```python
from build123d import *

# Parameters (mm, degrees)
SKETCH1_R           = 7.5
BOSS_EXTRUDE1_DEPTH = 230
SKETCH2_R           = 10
BOSS_EXTRUDE2_DEPTH = 5
SKETCH3_R           = 7.5
BOSS_EXTRUDE3_DEPTH = 10
CUT_EXTRUDE1_DEPTH  = 80
EXTRUDE_THIN1_DEPTH = 1.5


with BuildPart() as part:
    # Sketch1 → Boss-Extrude1 (new body)
    with BuildSketch(Plane.XY):
        Circle(SKETCH1_R)
    extrude(amount=BOSS_EXTRUDE1_DEPTH)

    # Sketch2 → Boss-Extrude2 (add)
    with BuildSketch(Plane.XY.offset(230)):
        Circle(SKETCH2_R)
    extrude(amount=BOSS_EXTRUDE2_DEPTH)

    # Sketch3 → Boss-Extrude3 (add)
    with BuildSketch(Plane.XY.offset(235)):
        Circle(SKETCH3_R)
    extrude(amount=BOSS_EXTRUDE3_DEPTH)

    # Sketch4 → Cut-Extrude1 (cut)
    with BuildSketch(Plane(origin=(0, 0, 0), x_dir=(-1, 0, 0), z_dir=(0, 0, -1))):
        with BuildLine():
            Line((-6.5, 3.741657387), (-6.5, -3.741657387))
            ThreePointArc((-6.5, -3.741657387), (-7.5, 0), (-6.5, 3.741657387))
        make_face()
        with BuildLine():
            Line((6.5, 3.741657387), (6.5, -3.741657387))
            ThreePointArc((6.5, -3.741657387), (7.5, 0), (6.5, 3.741657387))
        make_face()
    extrude(amount=-CUT_EXTRUDE1_DEPTH, mode=Mode.SUBTRACT)

    # Sketch5 → Extrude-Thin1 (add, symmetric)
    with BuildSketch(Plane(origin=(0, 0, 0), x_dir=(1, 0, 0), z_dir=(0, 1, 0))):
        with BuildLine():
            Line((-6, -245), (-6, -248))
            ThreePointArc((-6, -248), (0, -254), (6, -248))
            Line((6, -248), (6, -245))
            Line((6, -245), (16, -245))
            Line((16, -245), (16, -248))
            ThreePointArc((16, -248), (0, -264), (-16, -248))
            Line((-16, -248), (-16, -245))
            Line((-16, -245), (-6, -245))
        make_face()
    extrude(amount=EXTRUDE_THIN1_DEPTH, both=True)


solid = part.part
```
Check sheet for the modelled part. Datum: model origin and axes. Units: mm. A direction names the side the tool comes from. Round coordinates to 2 decimals unless told otherwise and drop trailing zeros. Loops run counter-clockwise (first coordinate to the right, second up) from the corner with the lowest first, then second, coordinate; pieces in that order, holes last. Notation, with made-up numbers: M 67,-30 L 92,-30 A13 cw 92,-11 Z; hole C 64,59.5 d2. An arc over 180 degrees is marked long. Answer as a JSON object with one key per item and string values.
1. Scan lines: line 1 (Y direction, x = 0.5, z = 26); line 2 (X direction, y = -6.5, z = 218); line 3 (Z direction, x = 4.5, y = 2.5). Record each from-to range of solid material in increasing order.
Reply:
{"line 1": "y = -7.48 to 7.48", "line 2": "x = -3.74 to 3.74", "line 3": "z = 0 to 245"}
2. Section check B-B (z = 198). Record the boundary of the cut face in (x, y).
Reply:
{"outline": "C 0,0 d15"}
3. Gauge pin test, flat ends, axial feed: P1, Ø1, axis at x = 0.5, z = 225.5, coming from the +Y side; P2, Ø1, axis at x = -11, y = 3.5, coming from the +Z side; P3, Ø6, axis at y = 0, z = 36, coming from the +X side; P4, Ø3.5, axis at x = 10, y = 0.5, coming from the -Z side. Record the tip position at first contact, or that the pin passes through.
Reply:
{"P1": "stops at y = 7.5", "P2": "passes through", "P3": "stops at x = 6.5", "P4": "stops at z = 230"}
4. Access from +Z, -Z, +X, -X, +Y, -Y to the whole of each face (thin tool, end or side, straight path). Record for faces 1 (the flat face through (0.2, -1.5, 254.4)), 2 (the flat face through (-6.5, 0, 39)), 3 (the flat face through (6.5, 0, 39)), 4 (the flat face through (0.2, 1.5, 254.4)).
Reply:
{"face 1": "+Z, +X, -X, -Y", "face 2": "-Z, -X, +Y, -Y", "face 3": "-Z, +X, +Y, -Y", "face 4": "+Z, +X, -X, +Y"}
5. Mould release check, pull along X, two halves, no side actions. Record for faces 5 (the flat face through (4, 7, 230)), 6 (the cylindrical face through (-7.493, 0.33, 113.39)), 7 (the cylindrical face through (0, 0, 254)): pulls with the +X half, pulls with the -X half, needs draft (parallel to the pull), parting line crosses it, or undercut.
Reply:
{"face 5": "needs draft", "face 6": "parting line crosses it", "face 7": "undercut"}
6. Section check A-A (x = 0). Record the boundary of the cut face in (y, z), plus the area to 3 significant figures.
Reply:
{"outline": "M -10,230 L -7.5,230 L -7.5,0 L 7.5,0 L 7.5,230 L 10,230 L 10,235 L 7.5,235 L 7.5,245 L -7.5,245 L -7.5,235 L -10,235 Z; M -1.5,254 L 1.5,254 L 1.5,264 L -1.5,264 Z", "area": "3,730 mm²"}
